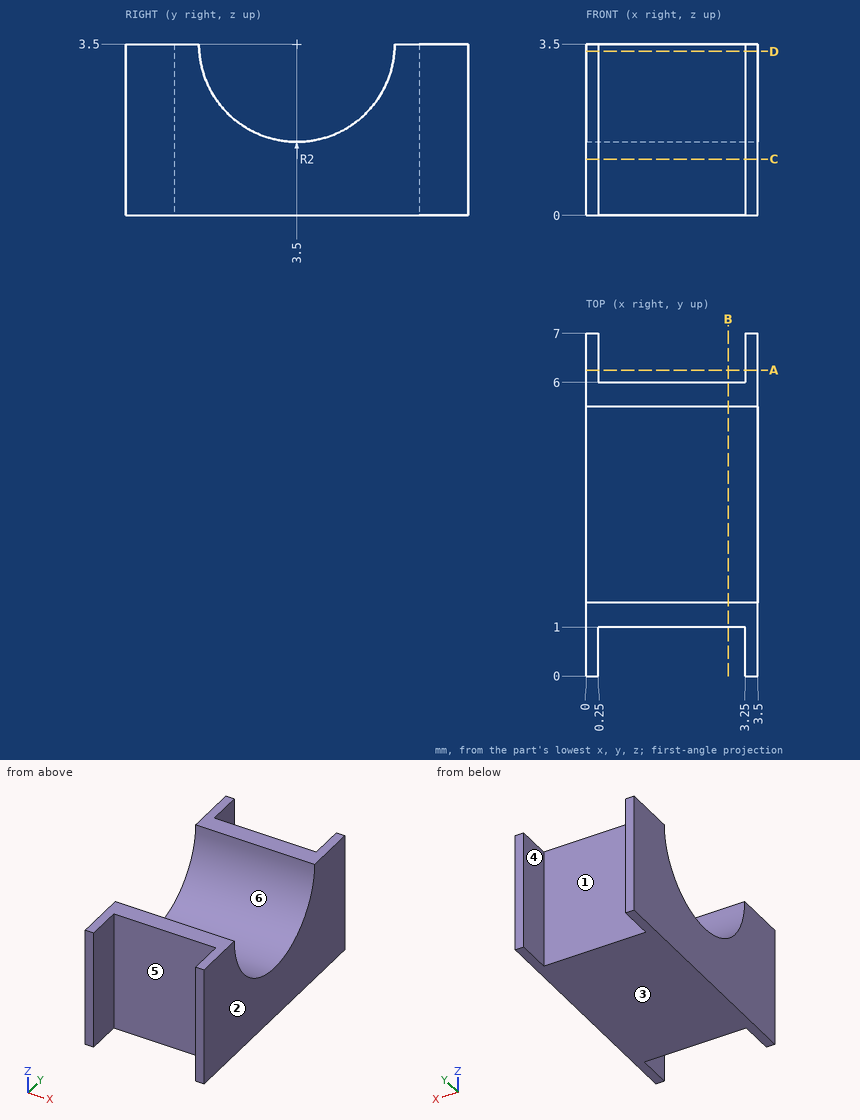
Source: three-view drawing plus pictorial views. Frame: mm from the lowest corner of the part. A direction names the side the tool comes from. Coordinates: 2 decimals unless noted, no trailing zeros. Order: outer loops, then holes, each group sorted by start corner. A loop starts at its lowest first (then second) coordinate and runs counter-clockwise, first axis right, second up. Notation, with made-up numbers: M -17.5,65.5 L 35.5,65.5 A33 ccw 35.5,103.5 Z; hole C -33.75,37 d9. An arc over 180 degrees is marked long. Answer in a Markdown table with one row per item.
(1) Section query A-A, the plane y = 6.25. Output: boundary loops of the cut face in (x, z).
Numbers:
| item | result |
|---|---|
| outline | M 0,0 L 0.25,0 L 0.25,3.5 L 0,3.5 Z; M 3.25,0 L 3.5,0 L 3.5,3.5 L 3.25,3.5 Z |
(2) Contact query for a flat-ended pin moving along its axis: pin 1 Ø1 at (x, z) = (2, 2.5) entering from +Y. Output: stop coordinate, or through.
Numbers:
| item | result |
|---|---|
| pin 1 | stops at y = 6 |
(3) Access query for the marked faces 4, 5 and 6. Directions: +Z, -Z, +X, -X, +Y, -Y. A direction counts if a zero-diameter tool reaches every point of the face in a straight line with its end or side. Return the directions, or none.
Numbers:
| item | result |
|---|---|
| face 4 | +Z, -Z, +Y |
| face 5 | +Z, -Z, -Y |
| face 6 | +Z, +X, -X |
(4) Section query D-D, the plane z = 3.35. Output: boundary loops of the cut face in (x, y), plus the area to 3 significant figures.
Numbers:
| item | result |
|---|---|
| outline | M 0,0 L 0.25,0 L 0.25,1 L 3.25,1 L 3.25,0 L 3.5,0 L 3.5,1.51 L 0,1.51 Z; M 0,5.49 L 3.5,5.49 L 3.5,7 L 3.25,7 L 3.25,6 L 0.25,6 L 0.25,7 L 0,7 Z |
| area | 4.54 mm^2 |
(5) Material intervals for line 1 (X direction, y = 0.5, z = 2.6); line 2 (Y direction, x = 1.6, z = 1); line 3 (Y direction, x = 0.3, z = 2.9), sorted ascending. Write a range as [from, to].
Numbers:
| item | result |
|---|---|
| line 1 | x = [0, 0.25], [3.25, 3.5] |
| line 2 | y = [1, 6] |
| line 3 | y = [1, 1.59], [5.41, 6] |
(6) Draft query along X for the marked faces 1, 2 and 3. Return one class per face: pulls with the +X half, pulls with the -X half, needs draft (parallel to the pull), parting line crosses it, or undercut.
Numbers:
| item | result |
|---|---|
| face 1 | undercut |
| face 2 | pulls with the +X half |
| face 3 | needs draft |
(7) Section query C-C, the plane z = 1.15. Output: boundary loops of the cut face in (x, y), plus the area to 3 significant figures.
Numbers:
| item | result |
|---|---|
| outline | M 0,0 L 0.25,0 L 0.25,1 L 3.25,1 L 3.25,0 L 3.5,0 L 3.5,7 L 3.25,7 L 3.25,6 L 0.25,6 L 0.25,7 L 0,7 Z |
| area | 18.5 mm^2 |
(8) Section query B-B, the plane x = 2.9. Output: boundary loops of the cut face in (y, z).
Numbers:
| item | result |
|---|---|
| outline | M 1,0 L 6,0 L 6,3.5 L 5.5,3.5 A2 cw 1.5,3.5 L 1,3.5 Z |
